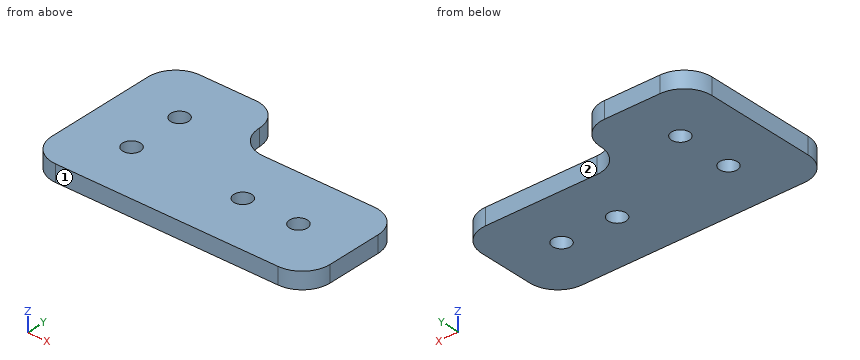
```python
from build123d import *

# Parameters (mm, degrees)
SKETCH_1_R      = 1.6
EXTRUDE_1_DEPTH = 3
FILLET_1_R      = 5


with BuildPart() as part:
    # 草图1 → 凸台-拉伸1 (new body)
    with BuildSketch(Plane.XY):
        Polygon((0, 0), (0, 30), (20, 30), (20, 20), (50, 20), (50, 0), align=None)
        with Locations((10, 20)):
            Circle(SKETCH_1_R, mode=Mode.SUBTRACT)
        with Locations((10, 10)):
            Circle(SKETCH_1_R, mode=Mode.SUBTRACT)
        with Locations((30, 10)):
            Circle(SKETCH_1_R, mode=Mode.SUBTRACT)
        with Locations((40, 10)):
            Circle(SKETCH_1_R, mode=Mode.SUBTRACT)
    extrude(amount=EXTRUDE_1_DEPTH)

    # 圆角1
    fillet_1_edges = [part.edges().sort_by_distance(p)[0] for p in [
        (0, 0, 1.5),
        (50, 0, 1.5),
        (50, 20, 1.5),
        (20, 20, 1.5),
        (20, 30, 1.5),
        (0, 30, 1.5),
    ]]
    fillet(fillet_1_edges, radius=FILLET_1_R - 0.0001)  # a hair under: the kernel refuses the full size


solid = part.part
```
The model under review builds one solid part; all positions refer to its coordinate system, in mm. Face numbers are marked on the shaded views. A direction names the side the tool comes from. Round coordinates to 2 decimals unless told otherwise and drop trailing zeros. Order: outer loops, then holes, each group sorted by start corner. A loop starts at its lowest first (then second) coordinate and runs counter-clockwise, first axis right, second up. Notation, with made-up numbers: (-16.75, 28) -> (30.25, 28) arc R17 cw to (30.25, 50) -> close; hole circle Ø3 at (32, 18.5). An arc over 180 degrees is marked (long way). One line per item, written item: value. Start each with the question number.
Q1. Wall thickness on line 1 (Y direction, x = 10, z = 1.55); line 2 (Y direction, x = 11, z = 0.6); line 3 (X direction, y = 11, z = 0.85): over which ranges is each line inside the solid? List them lowest first.
Q2. Clearance check with a flat-ended pin moving along its axis: pin 1 Ø0.9 at (x, z) = (34, 2) entering from +Y. State where the tip first meets the part, or that it passes through.
Q3. Take a section at D-D (x = 40). Write out the cut boundary in (y, z).
Q4. Machinability: for the marked faces 1 and 2, which of the approach directions +Z, -Z, +X, -X, +Y, -Y give a long, thin tool a straight path to every point of the face, cutting with its end or side? Answer none if there is none.
Q5. Take a section at A-A (z = 2.15). Count the separate pieces of the cut face and the enclosed holes in it, and give its area (3 significant figures).
Q6. Take a section at C-C (y = 10). Write out the cut boundary in (x, z).
Q7. Take a section at B-B (x = 10). Write out the cut boundary in (y, z).
Reported:
1. line 1: y = 0 to 8.4, 11.6 to 18.4, 21.6 to 30
1. line 2: y = 0 to 8.75, 11.25 to 18.75, 21.25 to 30
1. line 3: x = 0 to 8.75, 11.25 to 28.75, 31.25 to 38.75, 41.25 to 50
2. pin 1: stops at y = 20
3. outline: (0, 0) -> (8.4, 0) -> (8.4, 3) -> (0, 3) -> close; (11.6, 0) -> (20, 0) -> (20, 3) -> (11.6, 3) -> close
4. face 1: +Z, -Z, +X, -X, -Y
4. face 2: +Z, -Z, +X, +Y
5. separate pieces: 1
5. enclosed holes: 4
5. area: 1,150 mm2
6. outline: (0, 0) -> (8.4, 0) -> (8.4, 3) -> (0, 3) -> close; (11.6, 0) -> (28.4, 0) -> (28.4, 3) -> (11.6, 3) -> close; (31.6, 0) -> (38.4, 0) -> (38.4, 3) -> (31.6, 3) -> close; (41.6, 0) -> (50, 0) -> (50, 3) -> (41.6, 3) -> close
7. outline: (0, 0) -> (8.4, 0) -> (8.4, 3) -> (0, 3) -> close; (11.6, 0) -> (18.4, 0) -> (18.4, 3) -> (11.6, 3) -> close; (21.6, 0) -> (30, 0) -> (30, 3) -> (21.6, 3) -> close
